Autodesk Inventor part; units mm, degrees
ref_plane "YZ Plane" through (0, 0, 0) normal (1, 0, 0) x (0, 1, 0)
ref_plane "XZ Plane" through (0, 0, 0) normal (0, 1, 0) x (-1, 0, 0)
ref_plane "XY Plane" through (0, 0, 0) normal (0, 0, 1) x (1, 0, 0)
sketch "Náčrt1" plane through (0, 0, 0) normal (0, 1, 0) x (-1, 0, 0)
  line L0 (0, 0) -> (-9.5, 0)
  line L1 (-9.5, 0) -> (-9.5, -7)
  line L2 (-9.5, -7) -> (0, -7)
  line L3 (0, -7) -> (0, 0)
  dimension "d0" = 9.5
  dimension "d1" = 7
extrude "Vysunutí1" add sketch "Náčrt1" along normal blind 1
sketch "Náčrt2" plane through (0, 1, 0) normal (0, 1, 0) x (1, 0, 0)
  line L0 (1.1, 1.1) -> (8.4, 1.1)
  line L1 (8.4, 1.1) -> (8.4, 5.9)
  line L2 (8.4, 5.9) -> (1.1, 5.9)
  line L3 (1.1, 5.9) -> (1.1, 1.1)
  line L4 (9.5, 7) -> (0, 7)
  line L5 (0, 7) -> (0, 0)
  dimension "d4" = 7.3
  dimension "d5" = 4.8
  dimension "d6" = 1.1
  dimension "d7" = 1.1
extrude "Vysunutí2" add sketch "Náčrt2" along normal blind 3.5
chamfer "Zkosení1" distance 0.9 angle 45 4 edges at (1.1, 2.75, -5.9) (1.1, 2.75, -1.1) (8.4, 2.75, -1.1) (8.4, 2.75, -5.9)
sketch "Náčrt3" plane through (0, 0, 0) normal (0, 0, 1) x (1, 0, 0)
  point P0 (0, 0)
sketch "Náčrt4" plane through (0, 1, 0) normal (0, 1, 0) x (1, 0, 0)
  point P0 (0, 0)
properties part number "MiddleButton"
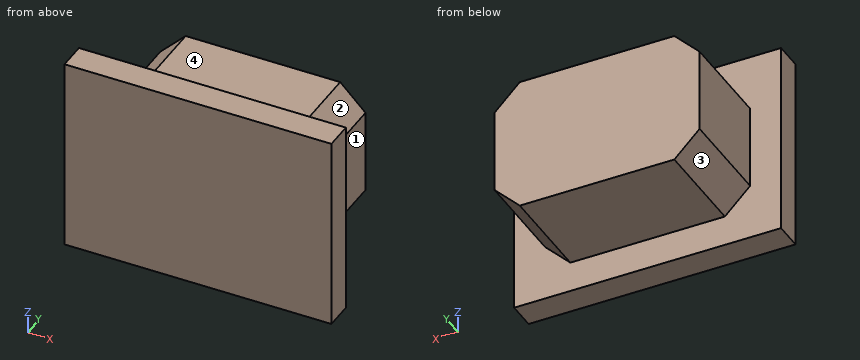
Could you check a few things on this model? Use its own coordinates, in mm. Face numbers are marked on the shaded views. A direction names the side the tool comes from. Round coordinates to 2 decimals unless told otherwise and drop trailing zeros. Loops run counter-clockwise (first coordinate to the right, second up) from the corner with the lowest first, then second, coordinate; pieces in that order, holes last. Notation, with made-up numbers: M 24.25,47.5 L 68.25,47.5 A37 cw 68.25,85.5 Z; hole C -20,-14.5 d2. An arc over 180 degrees is marked long. Put each result on its own line as item: value.
Q1. For pin 1 (0.9 mm diameter, centred on y = 2.5, z = -3.5, fed in from -X); pin 2 (1 mm diameter, centred on x = 4.5, y = 3.5, fed in from -Z); pin 3 (1 mm diameter, centred on x = 4.5, y = 3, fed in from +Z), each with a flat end and sliding along its axis, tell me the tip position at first contact or that it passes through.
Check result:
pin 1: x = 1.1
pin 2: z = -5.9
pin 3: z = -1.1
Q2. On a 3-axis mill with a long thin cutter (end or side, diameter ignored), from which of +Z, -Z, +X, -X, +Y, -Y can I reach the whole of each face in a straight line? I mean the marked faces 1, 2, 3 and 4. Say none if no direction works.
Check result:
face 1: +Z, -Z, +X, +Y
face 2: +Z, +X, +Y
face 3: -Z, -X, +Y
face 4: +Z, +X, -X, +Y
Q3. Imagine slicing it at A-A (x = 6). Write out the boundary of the cut face in (y, z).
Check result:
outline: M 0,-7 L 1,-7 L 1,-5.9 L 4.5,-5.9 L 4.5,-1.1 L 1,-1.1 L 1,0 L 0,0 Z
Q4. Imagine slicing it at B-B (y = 1.55). Write out the boundary of the cut face in (x, z), then the cut area to 3 significant figures.
Check result:
outline: M 1.1,-5 L 2,-5.9 L 7.5,-5.9 L 8.4,-5 L 8.4,-2 L 7.5,-1.1 L 2,-1.1 L 1.1,-2 Z
area: 33.4 mm2
Q5. I need wall thicknesses on probe 1 along X at (y, z) = (4, -2.25); probe 2 along Z at (x, y) = (4.75, 2.55); probe 3 along Y at (x, z) = (8.5, -5.25). Which ranges of each line are inside material? Lowest first, please.
Check result:
probe 1: 1.1 to 8.4
probe 2: -5.9 to -1.1
probe 3: 0 to 1
